Model file for the job. Use its own axes, mm. Round coordinates to 2 decimals unless told otherwise and drop trailing zeros. Loops run counter-clockwise (first coordinate to the right, second up) from the corner with the lowest first, then second, coordinate; pieces in that order, holes last. Notation, with made-up numbers: M 13,32.25 L 68,32.25 A28 ccw 68,65.25 Z; hole C -36.5,57 d7. An arc over 180 degrees is marked long. Use a Markdown table: item, result. Add a question column.
Q1. Cut at D-D (z = 3.25). Give the cut face in (x, y).
Q2. Cut at A-A (x = 0). Give the cut face in (y, z).
Q3. Cut at C-C (z = 0.75). Give the cut face in (x, y).
Q4. Probe line 1 (Z direction, x = 0, y = 42.5); line 2 (X direction, y = 12.5, z = -5.5); line 3 (Z direction, x = 4.25, y = 22.5). List the from-to ranges inside material, lowest first. Write a range as from..to.
Q5. Pin check, flat tips, straight feed: pin 1 (6 mm diameter, centred on y = 55, z = -2.5, fed in from +X); pin 2 (2 mm diameter, centred on y = 31, z = 3.5, fed in from +X). Stop position of each tip, or through.
Q6. Mould opens along Z. For faces 1 (the face through (0.33, 31.31, -2.52)), 2 (the face through (0, 0, 3)), 3 (the face through (-4.18, 31.31, 5.46)) say: +Z half, -Z half, draft (parallel to the pull), parting line (faces both ways), or undercut.
Autodesk Inventor part; units mm, degrees
ref_plane "YZ Plane" through (0, 0, 0) normal (1, 0, 0) x (0, 1, 0)
ref_plane "XZ Plane" through (0, 0, 0) normal (0, 1, 0) x (-1, 0, 0)
ref_plane "XY Plane" through (0, 0, 0) normal (0, 0, 1) x (1, 0, 0)
sketch "Sketch1" plane through (0, 0, 0) normal (0, 1, 0) x (-1, 0, 0)
  line L0 (-3.6662, 6.35) -> (3.6662, 6.35)
  line L1 (3.6662, 6.35) -> (7.3323, 0)
  line L2 (7.3323, 0) -> (3.6662, -6.35)
  line L3 (3.6662, -6.35) -> (-3.6662, -6.35)
  line L4 (-3.6662, -6.35) -> (-7.3323, 0)
  line L5 (-7.3323, 0) -> (-3.6662, 6.35)
  circle A0 centre (0, 0) radius 2.54
  dimension "d0" = 12.7
  dimension "d1" = 5.08
extrude "Extrusion1" add sketch "Sketch1" along normal blind 63.5
sketch "Sketch2" plane through (0, 63.5, 0) normal (0, 1, 0) x (1, 0, 0)
  line L0 (-3.6662, 6.35) -> (3.6662, 6.35)
  arc A0 (-1.5875, 6.35) -> (1.5875, 6.35) centre (0, 6.35) ccw
  line L1 (-1.5875, 6.35) -> (1.5875, 6.35)
  dimension "d4" = 1.5875
extrude "Extrusion2" cut sketch "Sketch2" against normal through all
pattern_circular "Circular Pattern1" count 6 over 360 about axis through (0, 0, 0) along (0, 1, 0) of "Extrusion2"
properties part number "UpperPlateStandoff" material "Aluminum-6061"
Checked values:
| question | item | result |
|---|---|---|
| 1 | outline | M -3.91,0 L 3.91,0 L 3.91,63.5 L -3.91,63.5 Z |
| 2 | outline | M 0,-4.76 L 63.5,-4.76 L 63.5,-2.54 L 0,-2.54 Z; M 0,2.54 L 63.5,2.54 L 63.5,4.76 L 0,4.76 Z |
| 3 | outline | M -6.9,0 L -2.43,0 L -2.43,63.5 L -6.9,63.5 Z; M 2.43,0 L 6.9,0 L 6.9,63.5 L 2.43,63.5 Z |
| 4 | line 1 | z = -4.76..-2.54, 2.54..4.76 |
| 4 | line 2 | x = -4.16..-1.34, 1.34..4.16 |
| 4 | line 3 | z = -5.34..-4.15, -2.2..2.2, 4.15..5.34 |
| 5 | pin 1 | stops at x = 7.33 |
| 5 | pin 2 | stops at x = 4.62 |
| 6 | face 1 | undercut |
| 6 | face 2 | draft |
| 6 | face 3 | +Z half |
